Geometry check sheet. Reference: the model listing, model coordinates, mm. Face numbers are marked on the shaded views. Round coordinates to 2 decimals unless told otherwise and drop trailing zeros. Write each loop counter-clockwise with the first axis right and the second up, starting at its lowest first coordinate (ties: lowest second). Pieces come first, ordered by that corner, then holes.
Item 1: Cross-section at A-A (x = 64). Enter the section's corners in (y, z), then the cut area to 3 significant figures.
Item 2: Depth check by flat-ended pin: P1, Ø1.4, axis at x = -32.5, z = 7, coming from the +Y side; P2, Ø1.5, axis at x = 10, z = -5, coming from the -Y side; P3, Ø3, axis at x = -109, z = -3.5, coming from the +Y side; P4, Ø5.5, axis at x = 65, z = -4.5, coming from the +Y side. Enter the tip coordinate at first touch or a pass-through.
Item 3: Scan lines: probe 1 along Z at (x, y) = (-21, -12); probe 2 along Z at (x, y) = (-37, -21); probe 3 along Y at (x, z) = (-73.5, 6.5). Record each from-to range of solid material in increasing order.
Item 4: Cross-section at B-B (y = -18). Enter the section's corners in (x, z).
Item 5: Cross-section at C-C (y = -4.5). Enter the section's corners in (x, z), then the cut area to 3 significant figures.
Item 6: Draft check along Z on the marked faces 1, 2 and 3. Enter one of: pulls with the +Z half, pulls with the -Z half, needs draft (parallel to the pull), parting line crosses it, or undercut.
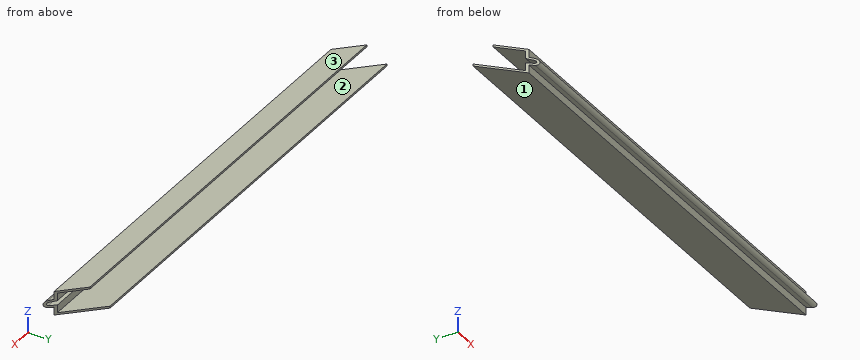
from build123d import *

# Parameters (mm, degrees)
BOSS_EXTRUDE1_DEPTH         = 152.4
CUT_FRONT_LEFT_BOTTOM_DEPTH = 16.24
CUT_FRONT_RIGHT_TOP_DEPTH   = 16.24


with BuildPart() as part:
    # Sketch1 → Boss-Extrude1 (new body, symmetric)
    with BuildSketch(Plane(origin=(0, 0, 0), x_dir=(0, 0, -1), z_dir=(1, 0, 0))):
        with BuildLine():
            Line((7.62, 0), (7.62, -21.844))
            Line((7.62, -21.844), (2.54, -21.844))
            Line((2.54, -21.844), (2.202186415, -24.247668555))
            ThreePointArc((2.202186415, -24.247668555), (0, -26.162), (-2.202186415, -24.247668555))
            Line((-2.202186415, -24.247668555), (-2.54, -21.844))
            Line((-2.54, -21.844), (-7.62, -21.844))
            Line((-7.62, -21.844), (-7.62, -7.874))
            Line((-7.62, -7.874), (-6.35, -7.874))
            Line((-6.35, -7.874), (-6.35, -20.574))
            Line((-6.35, -20.574), (-1.436005843, -20.574))
            Line((-1.436005843, -20.574), (-0.944545968, -24.070918717))
            ThreePointArc((-0.944545968, -24.070918717), (0, -24.892), (0.944545968, -24.070918717))
            Line((0.944545968, -24.070918717), (1.436005843, -20.574))
            Line((1.436005843, -20.574), (6.35, -20.574))
            Line((6.35, -20.574), (6.35, 0))
            Line((6.35, 0), (7.62, 0))
        make_face()
    extrude(amount=BOSS_EXTRUDE1_DEPTH, both=True)

    # Sketch12 → Cut-Front-Left-Bottom (cut, through all)
    with BuildSketch(Plane.XY.offset(7.62)):
        Polygon((-152.4, 0), (-126.238, -26.162), (-152.4, -26.162), align=None)
    extrude(amount=-CUT_FRONT_LEFT_BOTTOM_DEPTH, mode=Mode.SUBTRACT)

    # Sketch7 → Cut-Front-Right-Top (cut, through all)
    with BuildSketch(Plane.XY.offset(7.62)):
        Polygon((152.4, -26.162), (126.238, 0), (152.4, 0), align=None)
    extrude(amount=-CUT_FRONT_RIGHT_TOP_DEPTH, mode=Mode.SUBTRACT)


solid = part.part
Resolved:
1. outline: (-24.25, -2.2) - (-21.84, -2.54) - (-21.84, -7.62) - (0, -7.62) - (0, -6.35) - (-20.57, -6.35) - (-20.57, -1.44) - (-24.07, -0.94) arc R0.95 cw to (-24.07, 0.94) - (-20.57, 1.44) - (-20.57, 6.35) - (-7.87, 6.35) - (-7.87, 7.62) - (-21.84, 7.62) - (-21.84, 2.54) - (-24.25, 2.2) arc R2.22 ccw to start
1. area: 69.9 mm2
2. P1: stops at y = -7.87
2. P2: stops at y = -21.84
2. P3: stops at y = -20.57
2. P4: stops at y = 0
3. probe 1: z = -7.62 to -6.35, 6.35 to 7.62
3. probe 2: z = -7.62 to -1.38, 1.38 to 7.62
3. probe 3: y = -21.84 to -7.87
4. outline: (-134.4, -7.62) - (144.24, -7.62) - (144.24, -6.35) - (-134.4, -6.35) - close; (-134.4, 6.35) - (144.24, 6.35) - (144.24, 7.62) - (-134.4, 7.62) - close
5. outline: (-147.9, -7.62) - (130.74, -7.62) - (130.74, -6.35) - (-147.9, -6.35) - close
5. area: 354 mm2
6. face 1: pulls with the -Z half
6. face 2: undercut
6. face 3: pulls with the +Z half
